```python
from build123d import *

# Parameters (mm, degrees)
F0_W     = 127
F0_H     = 88.9
F0_R     = 6.35
F0_R_2   = 88.9
F1_DEPTH = 9.525
F3_DEPTH = 38.1
F5_DEPTH = 38.1


with BuildPart() as f1:
    # F0 (on Top) → F1 (new body)
    with BuildSketch(Plane.XY):
        with Locations((63.5, 44.45)):
            Rectangle(F0_W, F0_H)
        with Locations((12.7, 27.647039)):
            Circle(F0_R, mode=Mode.SUBTRACT)
        with Locations((114.3, 27.647039)):
            Circle(F0_R, mode=Mode.SUBTRACT)
        Polygon((127, 0), (0, 0), (-152.4, 0), (-152.4, -304.8), (279.4, -304.8), (279.4, 0), align=None)
        with Locations((63.5, -177.8)):
            Circle(F0_R_2, mode=Mode.SUBTRACT)
    extrude(amount=F1_DEPTH)

    # F2 (on face) → F3 (join)
    with BuildSketch(Plane(origin=(-152.4, 0, 0), x_dir=(0, -1, 0), z_dir=(-1, 0, 0))):
        Polygon((0.009177, -800.095136), (304.8, 0), (266.7, 0), (-38.018486, -799.905247), align=None)
    extrude(amount=-F3_DEPTH)

    # F4 (on face) → F5 (join)
    with BuildSketch(Plane.YZ.offset(279.4)):
        Polygon((-266.7, 0), (-304.8, 0), (-0.016334, -800.048764), (38.018486, -799.905247), align=None)
    extrude(amount=-F5_DEPTH)


solid = f1.part
```
Input: part model. Units: mm. Frame: model coordinates. A direction names the side the tool comes from. Coordinates: 2 decimals unless noted, no trailing zeros. Write each loop counter-clockwise with the first axis right and the second up, starting at its lowest first coordinate (ties: lowest second). Pieces come first, ordered by that corner, then holes. Notation, with made-up numbers: (41.5, 78.5) -> (71.5, 78.5) arc R9 ccw to (71.5, 93.5) -> close; hole circle Ø9 at (81, 14). An arc over 180 degrees is marked (long way). Write each question's results on one line, items separated by ' | '.
Item 1: Set-up query: faces 5 (the flat face through (60, -61, 0)), 6 (the flat face through (-133.617, -116.474, -394.353)), 7 (the flat face through (241.3, -134, -398)). Return all of +Z, -Z, +X, -X, +Y, -Y with unobstructed straight access to the full face (end or side cutting, diameter ignored); none if empty.
Conclusion:
face 5: +Y | face 6: +X, -X, +Y | face 7: -Z, +Y, -Y
Item 2: Mould query, pull axis Z, two halves, no side actions, for faces 1 (the flat face through (60, -61, 9.525)), 2 (the cylindrical face through (104.52, -256.67, 4.7)), 3 (the flat face through (-133.62, -150.27, -405.65)), 4 (the flat face through (260.62, -112.21, -405.55)). Classes: +Z half, -Z half, draft (parallel to the pull), parting line (faces both ways), or undercut.
Conclusion:
face 1: +Z half | face 2: draft | face 3: -Z half | face 4: undercut
Item 3: Section query C-C on z = -206. Return loops of the section in (x, y).
Conclusion:
outline: (-152.4, -226.33) -> (-114.3, -226.33) -> (-114.3, -188.23) -> (-152.4, -188.23) -> close; (241.3, -226.32) -> (279.4, -226.32) -> (279.4, -188.23) -> (241.3, -188.23) -> close
Item 4: Section query A-A on x = 63.5. Return loops of the section in (y, z) (3 decimals).
Conclusion:
outline: (-304.8, 0) -> (-266.7, 0) -> (-266.7, 9.525) -> (-304.8, 9.525) -> close; (-88.9, 0) -> (88.9, 0) -> (88.9, 9.525) -> (-88.9, 9.525) -> close
Item 5: Section query B-B on y = -177.8. Return loops of the section in (x, z) (3 decimals), plus the area to 3 significant figures.
Conclusion:
outline: (-152.4, -333.383) -> (-114.3, -333.383) -> (-114.3, -233.368) -> (-152.4, -233.368) -> close; (-152.4, 0) -> (-25.4, 0) -> (-25.4, 9.525) -> (-152.4, 9.525) -> close; (152.4, 0) -> (279.4, 0) -> (279.4, 9.525) -> (152.4, 9.525) -> close; (241.3, -333.372) -> (279.4, -333.372) -> (279.4, -233.368) -> (241.3, -233.368) -> close | area: 10,000 mm^2
Item 6: Material intervals for probe 1 along X at (y, z) = (-133, -443.5); probe 2 along Y at (x, z) = (114, 4); probe 3 along Y at (x, z) = (12, 6), sorted ascending.
Conclusion:
probe 1: x = -152.4 to -114.3, 241.3 to 279.4 | probe 2: y = -304.8 to -250.96, -104.64 to 21.3, 33.99 to 88.9 | probe 3: y = -304.8 to -250.26, -105.34 to 21.34, 33.96 to 88.9
Item 7: Pin query (flat end, axial travel): pin 1 Ø10 at (x, y) = (112, -57) entering from -Z; pin 2 Ø3 at (x, z) = (-45.5, 3.5) entering from +Y; pin 3 Ø10.5 at (y, z) = (25.5, 4.5) entering from +X; pin 4 Ø16.5 at (x, y) = (114.3, 27.65) entering from +Z (3 decimals). Return the tip coordinate at first contact, or that it passes through.
Conclusion:
pin 1: stops at z = 0 | pin 2: stops at y = 0 | pin 3: stops at x = 127 | pin 4: stops at z = 9.525
Item 8: Section query D-D on y = -37.5. Return loops of the section in (x, z) (3 decimals), plus the area to 3 significant figures.
Conclusion:
outline: (-152.4, -701.679) -> (-114.3, -701.679) -> (-114.3, -601.664) -> (-152.4, -601.664) -> close; (-152.4, 0) -> (279.4, 0) -> (279.4, 9.525) -> (-152.4, 9.525) -> close; (241.3, -701.655) -> (279.4, -701.655) -> (279.4, -601.664) -> (241.3, -601.664) -> close | area: 11,700 mm^2
